Verification items for the finished model (mm, model axes). A direction names the side the tool comes from. Coordinates: 2 decimals unless noted, no trailing zeros. Order: outer loops, then holes, each group sorted by start corner. A loop starts at its lowest first (then second) coordinate and runs counter-clockwise, first axis right, second up. Notation, with made-up numbers: (68.5, 38.25) -> (76.5, 38.25) arc R10 ccw to (76.5, 54.25) -> close; hole circle Ø8 at (38, 67). An arc over 180 degrees is marked (long way). Answer as CSV lines item,"result".
```python
from build123d import *

# Parameters (mm, degrees)
F0_W           = 24
F0_H           = 7.5
F1_DEPTH       = 3
F2_D           = 3.4
F2_CSINK_D     = 6.6
F2_CSINK_ANGLE = 90
F3_W           = 9.4
F3_H           = 3
F4_DEPTH       = 10.5
F5_W           = 9.4
F5_H           = 2
F6_DEPTH       = 4


with BuildPart() as f1:
    # F0 (on Front) → F1 (new body)
    with BuildSketch(Plane.XZ):
        Rectangle(F0_W, F0_H)
    extrude(amount=F1_DEPTH)

    # F2 (through all)
    with Locations(Plane(origin=(0, 0, 0), x_dir=(1, 0, 0), z_dir=(0, 1, 0))):
        with Locations((-8.5, 0), (8.5, 0)):
            CounterSinkHole(F2_D / 2, F2_CSINK_D / 2, counter_sink_angle=F2_CSINK_ANGLE)

    # F3 (on face) → F4 (join)
    with BuildSketch(Plane.XZ):
        with Locations((0, 2.25)):
            Rectangle(F3_W, F3_H)
    extrude(amount=-F4_DEPTH)

    # F5 (on face) → F6 (join)
    with BuildSketch(Plane(origin=(0, 0, 0.75), x_dir=(1, 0, 0), z_dir=(0, 0, -1))):
        with Locations((0, -9.5)):
            Rectangle(F5_W, F5_H)
    extrude(amount=F6_DEPTH)


solid = f1.part
```
Item 1: Section check A-A, the plane x = -8.5. Record the boundary of the cut face in (y, z).
Answer list:
outline,"(-3, -3.75) -> (0, -3.75) -> (0, -3.3) -> (-1.6, -1.7) -> (-3, -1.7) -> close; (-3, 1.7) -> (-1.6, 1.7) -> (0, 3.3) -> (0, 3.75) -> (-3, 3.75) -> close"
Item 2: Release check for a two-part mould opening along X. For faces 1 (the flat face through (-12, -1, 0)), 2 (the cylindrical face through (-7.15, -2.31, 1.03)), 3 (the cylindrical face through (9.85, -2.31, 1.03)), 4 (the flat face through (0, 4, 0.75)) record: +X half, -X half, draft (parallel to the pull), parting line (faces both ways), or undercut.
Answer list:
face 1,"-X half"
face 2,"undercut"
face 3,"undercut"
face 4,"draft"
Item 3: Thickness scan on line 1 (Y direction, x = -4, z = -2.5); line 2 (X direction, y = -0.25, z = 0.5); line 3 (Z direction, x = 8.5, y = -2.65). Record the ranges inside material, lowest first.
Answer list:
line 1,"-3 to 0, 8.5 to 10.5"
line 2,"-12 to -11.51, -5.49 to 5.49, 11.51 to 12"
line 3,"-3.75 to -1.7, 1.7 to 3.75"
Item 4: Depth check by flat-ended pin: pin 1 Ø2 at (x, y) = (-2, 10) entering from -Z; pin 2 Ø4 at (y, z) = (4.5, 2) entering from -X; pin 3 Ø2 at (y, z) = (5.5, 1.5) entering from +X. Enter the tip coordinate at first touch or a pass-through.
Answer list:
pin 1,"z = -3.25"
pin 2,"x = -4.7"
pin 3,"x = 4.7"
Item 5: Section check B-B, the plane z = 0. Record the boundary of the cut face in (x, y).
Answer list:
outline,"(-12, -3) -> (-10.2, -3) -> (-10.2, -1.6) -> (-11.8, 0) -> (-12, 0) -> close; (-6.8, -3) -> (6.8, -3) -> (6.8, -1.6) -> (5.2, 0) -> (-5.2, 0) -> (-6.8, -1.6) -> close; (-4.7, 8.5) -> (4.7, 8.5) -> (4.7, 10.5) -> (-4.7, 10.5) -> close; (10.2, -3) -> (12, -3) -> (12, 0) -> (11.8, 0) -> (10.2, -1.6) -> close"
Item 6: Section check C-C, the plane x = -3.25. Record the boundary of the cut face in (y, z), plus the area to 3 significant figures.
Answer list:
outline,"(-3, -3.75) -> (0, -3.75) -> (0, 0.75) -> (8.5, 0.75) -> (8.5, -3.25) -> (10.5, -3.25) -> (10.5, 3.75) -> (-3, 3.75) -> close"
area,"62.0 mm2"
Item 7: Section check D-D, the plane y = 3.5. Record the boundary of the cut face in (x, z).
Answer list:
outline,"(-4.7, 0.75) -> (4.7, 0.75) -> (4.7, 3.75) -> (-4.7, 3.75) -> close"
Item 8: Tool access check on faces 5 (the flat face through (-4.7, 6, 2)), 6 (the flat face through (0, 0, -1)), 7 (the flat face through (0, 8.5, -1)). Record the directions out of +Z, -Z, +X, -X, +Y, -Y that give a thin tool (end or side, any length) a straight path to the whole face; none if there is none.
Answer list:
face 5,"+Z, -Z, -X, +Y"
face 6,"-Z"
face 7,"-Z, +X, -X"
